Model file for the job. Use its own axes, mm. Coordinates: 2 decimals unless noted, no trailing zeros. Write each loop counter-clockwise with the first axis right and the second up, starting at its lowest first coordinate (ties: lowest second). Pieces come first, ordered by that corner, then holes. Notation, with made-up numbers: M -37.5,60.5 L 8.5,60.5 A28 cw 8.5,82.5 Z; hole C 11.5,-25.5 d2. An arc over 180 degrees is marked long. Put each result on its own line as item: value. Start each with the question number.
Q1. Drill centre line: line 1 along Z through (x, y) = (8.5, 9.5). Where is it in solid material? Low to high.
Q2. Cut at A-A (x = -14). Write the cut outline in (y, z).
Q3. Drop a flat-ended pin along its axis: pin 1 (2 mm diameter, centred on x = 11, y = 2, fed in from -Z). Give the stop position or say it passes through.
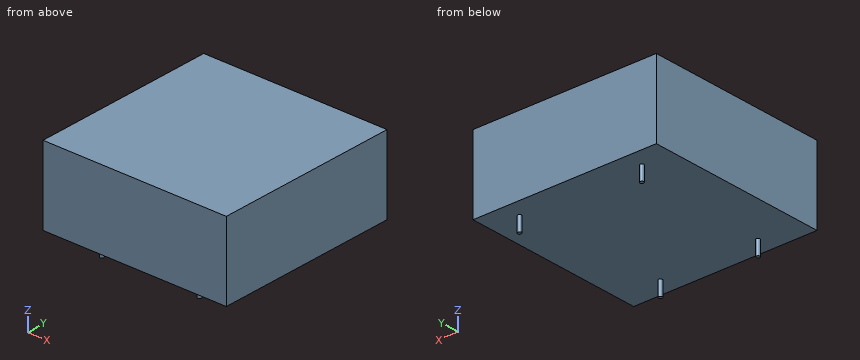
Autodesk Inventor part; units mm, degrees
ref_plane "YZ Plane" through (0, 0, 0) normal (1, 0, 0) x (0, 1, 0)
ref_plane "XZ Plane" through (0, 0, 0) normal (0, 1, 0) x (-1, 0, 0)
ref_plane "XY Plane" through (0, 0, 0) normal (0, 0, 1) x (1, 0, 0)
sketch "Skizze1" plane through (0, 0, 0) normal (0, 0, 1) x (1, 0, 0)
  line L0 (-19.05, 19.05) -> (19.05, 19.05)
  line L1 (19.05, 19.05) -> (19.05, -19.05)
  line L2 (19.05, -19.05) -> (-19.05, -19.05)
  line L3 (-19.05, -19.05) -> (-19.05, 19.05)
  line L4 (-19.05, 19.05) -> (19.05, -19.05) construction
  point P0 (0, 0)
  point P1 (0, 0)
  dimension "d0" = 38.1
  dimension "d1" = 38.1
extrude "Extrusion1" add sketch "Skizze1" along normal mid plane 16
sketch "Skizze2" plane through (0, 0, -8) normal (0, 0, -1) x (-1, 0, 0)
  line L0 (19.05, 19.05) -> (-19.05, 19.05) construction
  line L1 (-19.05, 19.05) -> (-19.05, -19.05) construction
  line L2 (-19.05, -19.05) -> (19.05, -19.05) construction
  line L3 (19.05, -19.05) -> (19.05, 19.05) construction
  line L4 (-19.05, -19.05) -> (-19.05, 19.05) construction
  line L5 (-19.05, -19.05) -> (-19.05, -15.24) construction
  line L6 (19.05, -19.05) -> (-19.05, -19.05) construction
  line L7 (19.05, -19.05) -> (19.05, -15.24) construction
  line L8 (19.05, 19.05) -> (19.05, -19.05) construction
  line L9 (-19.05, -15.24) -> (-10.16, -15.24) construction
  line L10 (19.05, -15.24) -> (10.16, -15.24) construction
  line L11 (-19.05, 19.05) -> (19.05, 19.05) construction
  line L12 (-19.05, 19.05) -> (-19.05, 15.24) construction
  line L13 (-19.05, 15.24) -> (-12.7, 15.24) construction
  line L14 (19.05, 19.05) -> (19.05, 15.24) construction
  line L15 (19.05, 15.24) -> (12.7, 15.24) construction
  circle A0 centre (-10.16, -15.24) radius 0.395
  circle A1 centre (-12.7, 15.24) radius 0.395
  circle A2 centre (12.7, 15.24) radius 0.395
  circle A3 centre (10.16, -15.24) radius 0.395
  point P0 (0, 0)
  dimension "d4" = 3.81
  dimension "d5" = 3.81
  dimension "d8" = 8.89
  dimension "d9" = 8.89
  dimension "d10" = 3.81
  dimension "d11" = 6.35
  dimension "d12" = 3.81
  dimension "d13" = 6.35
  dimension "d14" = 0.79
  dimension "d15" = 0.79
  dimension "d16" = 0.79
  dimension "d17" = 0.79
extrude "Extrusion4" add sketch "Skizze2" along normal blind 5.08
sketch "Skizze3" plane through (10.16, -15.24, -13.08) normal (0, 0, -1) x (-1, 0, 0)
  circle A0 centre (0, 0) radius 0.395
  circle A1 centre (20.32, 0) radius 0.395
  circle A2 centre (22.86, 30.48) radius 0.395
  circle A3 centre (-2.54, 30.48) radius 0.395
  point P0 (10.16, 15.24)
extrude "Extrusion5" cut sketch "Skizze3" against normal blind 2
properties part number "DC DC converter (M1730CQEA06065)"
Computed values:
1. line 1: -8 to 8
2. outline: M -19.05,-8 L 19.05,-8 L 19.05,8 L -19.05,8 Z
3. pin 1: z = -8
